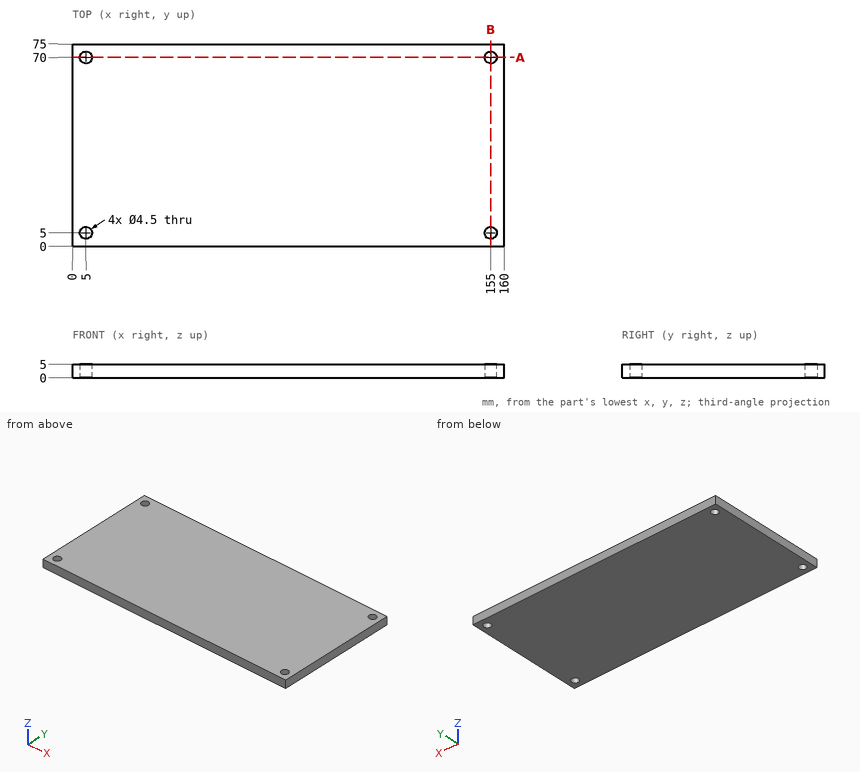
Geometry check sheet. Reference: drawing and pictorial views, mm from the part's lowest x, y, z. Give positions to 0.01 mm unless a question says otherwise; leave off trailing zeros. Loops run counter-clockwise (first coordinate to the right, second up) from the corner with the lowest first, then second, coordinate; pieces in that order, holes last. Notation, with made-up numbers: (-7, 62) - (33, 62) arc R18 ccw to (33, 76) - close; hole circle Ø10 at (84.5, 77.5). An arc over 180 degrees is marked (long way). Use CSV: the item, a comma, the result in double quotes. Start each with the question number.
Q1. Scan lines: probe 1 along Y at (x, z) = (5, 1.45); probe 2 along X at (y, z) = (5, 1.75). Record each from-to range of solid material in increasing order. Write a range as from..to.
Q2. Section check A-A, the plane y = 70. Record the cut outline in (x, z), and give its area (3 significant figures).
Q3. Section check B-B, the plane x = 155. Record the cut outline in (y, z).
Q4. Go/stop test with flat-tipped pins: pin 1 Ø5 at (x, y) = (155, 5) entering from -Z; pin 2 Ø3.5 at (x, y) = (155, 70) entering from -Z. Record where each tip stops, or that it passes through.
Findings below:
1,probe 1,"y = 0..2.75, 7.25..67.75, 72.25..75"
1,probe 2,"x = 0..2.75, 7.25..152.75, 157.25..160"
2,outline,"(0, 0) - (2.75, 0) - (2.75, 5) - (0, 5) - close; (7.25, 0) - (152.75, 0) - (152.75, 5) - (7.25, 5) - close; (157.25, 0) - (160, 0) - (160, 5) - (157.25, 5) - close"
2,area,"755 mm^2"
3,outline,"(0, 0) - (2.75, 0) - (2.75, 5) - (0, 5) - close; (7.25, 0) - (67.75, 0) - (67.75, 5) - (7.25, 5) - close; (72.25, 0) - (75, 0) - (75, 5) - (72.25, 5) - close"
4,pin 1,"stops at z = 0"
4,pin 2,"passes through"
